Job drawing, mm, ordinate dimensions from the low corner. One solid piece. A direction names the side the tool comes from. Coordinates: 2 decimals unless noted, no trailing zeros. Order: outer loops, then holes, each group sorted by start corner. A loop starts at its lowest first (then second) coordinate and runs counter-clockwise, first axis right, second up. Notation, with made-up numbers: (18.5, 65) - (58.5, 65) arc R27 ccw to (58.5, 102) - close; hole circle Ø4 at (-38.5, 48). An arc over 180 degrees is marked (long way). Use a Markdown table: item, result. Add a question column.
1) Tool access for the marked faces 1, 2 and 3: list every direction of +Z, -Z, +X, -X, +Y, -Y with a clear straight run to the whole face (end or side of a thin tool).
2) Drop flat-ended pins along their axis: P1, Ø6, axis at x = 21.5, y = 19, coming from the +Z side; P2, Ø3, axis at x = 21, z = 28, coming from the -Y side; P3, Ø1.5, axis at x = 27.5, z = 15.5, coming from the +Y side; P4, Ø10, axis at y = 13, z = 14, coming from the +X side. Give the stop position or say it passes through.
3) Two-plate mould, pull along Z, no slides. Class the marked faces 4, 5, 6 and 7: +Z half, -Z half, draft (parallel to the pull), parting line (faces both ways), or undercut.
4) Saw through at D-D on x = 37.5. List the corners of the cut face in (y, z), then the cut area to 3 significant figures.
5) Wall check: L1, parallel to Y at x = 25, z = 12.5; L2, parallel to Z at x = 15, y = 42; L3, parallel to Z at x = 48, y = 31.5. Give the ranges that are in metal, low to high. Write a range as [from, to].
6) Saw through at A-A on y = 25. List the corners of the cut face in (x, z).
7) Saw through at C-C on z = 6.5. List the corners of the cut face in (x, y), then the cut area to 3 significant figures.
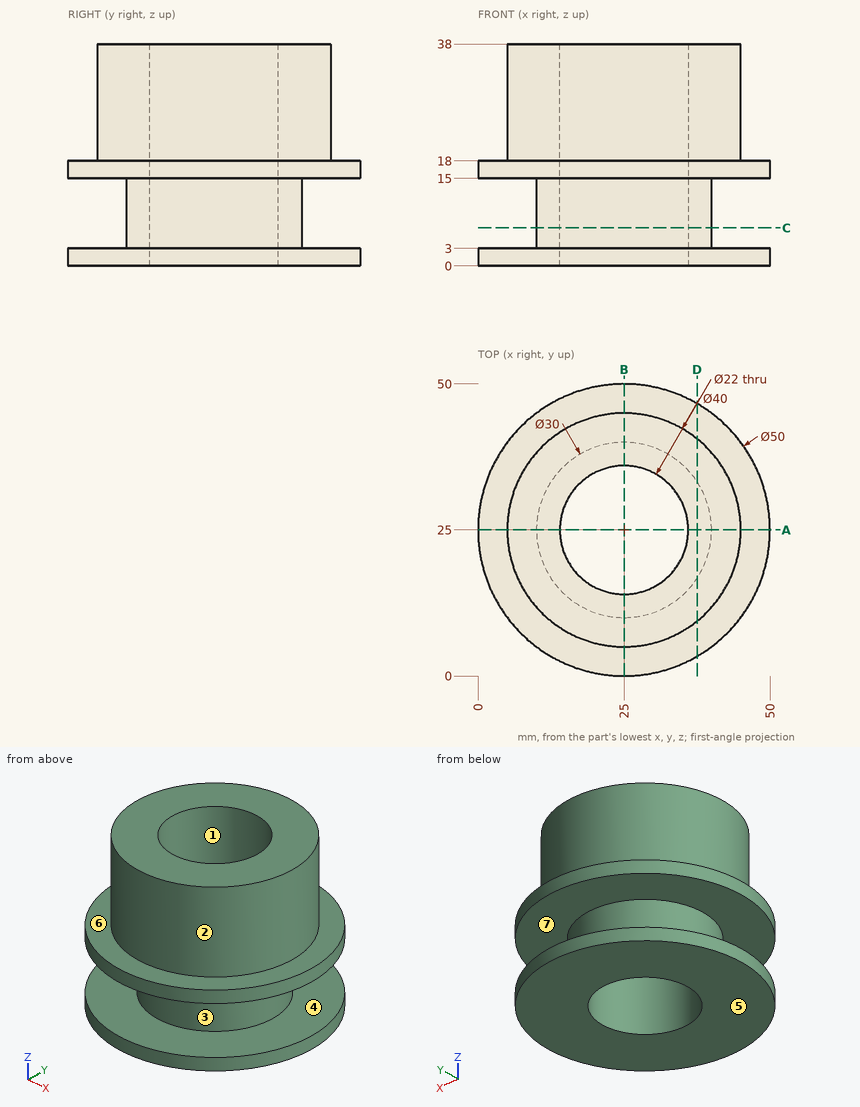
Results are:
| question | item | result |
|---|---|---|
| 1 | face 1 | +Z, -Z |
| 1 | face 2 | +Z |
| 1 | face 3 | none |
| 2 | P1 | through |
| 2 | P2 | y = 5.16 |
| 2 | P3 | y = 49.94 |
| 2 | P4 | x = 48.97 |
| 3 | face 4 | undercut |
| 3 | face 5 | -Z half |
| 3 | face 6 | +Z half |
| 3 | face 7 | undercut |
| 4 | outline | (3.35, 0) - (46.65, 0) - (46.65, 3) - (33.29, 3) - (33.29, 15) - (46.65, 15) - (46.65, 18) - (40.61, 18) - (40.61, 38) - (9.39, 38) - (9.39, 18) - (3.35, 18) - (3.35, 15) - (16.71, 15) - (16.71, 3) - (3.35, 3) - close |
| 4 | area | 1,080 mm2 |
| 5 | L1 | [10, 14], [36, 40] |
| 5 | L2 | [0, 3], [15, 38] |
| 5 | L3 | [0, 3], [15, 18] |
| 6 | outline | (0, 0) - (14, 0) - (14, 38) - (5, 38) - (5, 18) - (0, 18) - (0, 15) - (10, 15) - (10, 3) - (0, 3) - close; (36, 0) - (50, 0) - (50, 3) - (40, 3) - (40, 15) - (50, 15) - (50, 18) - (45, 18) - (45, 38) - (36, 38) - close |
| 7 | outline | circle Ø30 at (25, 25); hole circle Ø22 at (25, 25) |
| 7 | area | 327 mm2 |
